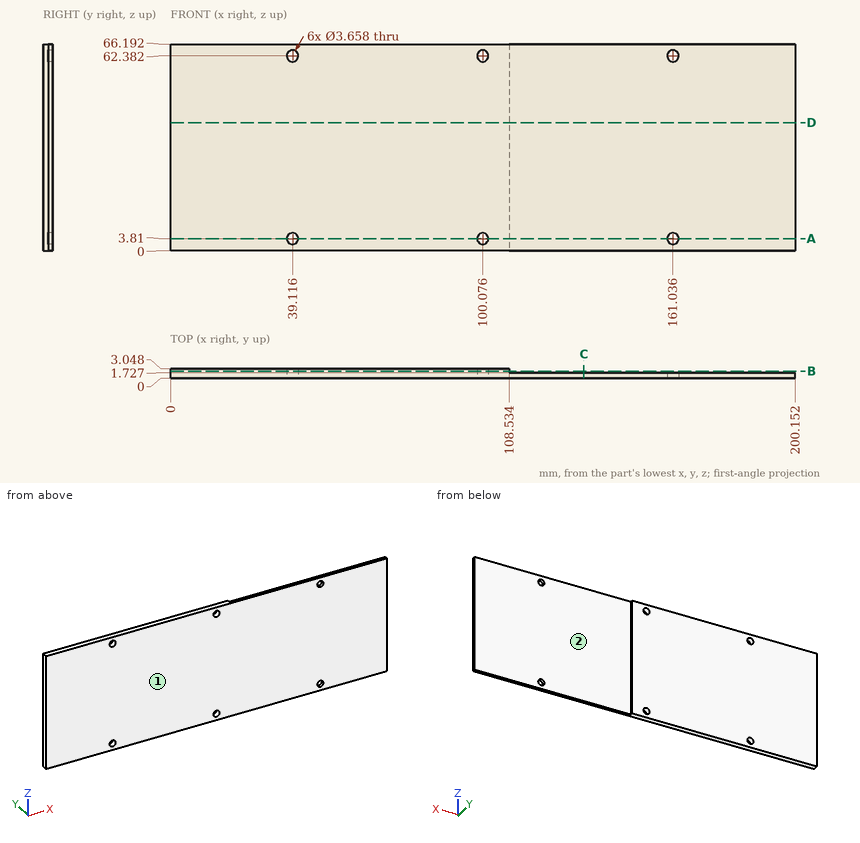
Drawing for the job (mm, zero at the part's lowest x, y, z). A direction names the side the tool comes from. Coordinates: 2 decimals unless noted, no trailing zeros. Order: outer loops, then holes, each group sorted by start corner. A loop starts at its lowest first (then second) coordinate and runs counter-clockwise, first axis right, second up. Notation, with made-up numbers: (17, 39) -> (40, 39) arc R31 cw to (40, 65) -> close; hole circle Ø7 at (6.5, -39.75). An arc over 180 degrees is marked (long way). Return JSON: item names as keys, results as strings.
Item 1: 3-axis set-ups, long thin cutter, end or side, ignore diameter. For the marked faces 1 and 2: which of +Z, -Z, +X, -X, +Y, -Y reach the whole face in a straight line?
Model answer:
{"face 1": "+Z, -Z, +X, -X, -Y", "face 2": "+Z, -Z, +X, +Y"}
Item 2: Wall check: line 1 along X through (y, z) = (0.9, 3.81) (1 decimal); line 2 along X through (y, z) = (1.8, 63) (1 decimal); line 3 along Z through (x, y) = (101.5, 0.35) (1 decimal). Give the ranges that are in metal, low to high. Write a range as from..to.
Model answer:
{"line 1": "x = 0..37.3, 40.9..98.2, 101.9..159.2, 162.9..200.2", "line 2": "x = 0..37.4, 40.8..98.4, 101.8..108.5", "line 3": "z = 0..2.7, 5..61.2, 63.5..66.2"}
Item 3: Slice it at A-A (z = 3.81). Write the cut outline in (x, y) (1 decimal).
Model answer:
{"outline": "(0, 0) -> (37.3, 0) -> (37.3, 3) -> (0, 3) -> close; (40.9, 0) -> (98.2, 0) -> (98.2, 3) -> (40.9, 3) -> close; (101.9, 0) -> (159.2, 0) -> (159.2, 1.7) -> (108.5, 1.7) -> (108.5, 3) -> (101.9, 3) -> close; (162.9, 0) -> (200.2, 0) -> (200.2, 1.7) -> (162.9, 1.7) -> close"}
Item 4: Slice it at C-C (x = 132.5). Write the cut outline in (y, z), then the cut area to 3 significant figures.
Model answer:
{"outline": "(0, 0) -> (1.73, 0) -> (1.73, 66.19) -> (0, 66.19) -> close", "area": "114 mm²"}
Item 5: Slice it at B-B (y = 2.2). Write the cut outline in (x, z) (1 decimal), then the cut area to 3 significant figures.
Model answer:
{"outline": "(0, 0) -> (108.5, 0) -> (108.5, 66.2) -> (0, 66.2) -> close; hole circle Ø3.7 at (39.1, 3.8); hole circle Ø3.7 at (39.1, 62.4); hole circle Ø3.7 at (100.1, 3.8); hole circle Ø3.7 at (100.1, 62.4)", "area": "7,140 mm²"}
Item 6: Pin check, flat tips, straight feed: P1, Ø1, axis at y = 2, z = 45.5, coming from the +X side; P2, Ø6, axis at x = 161.04, z = 62.38, coming from the +Y side; P3, Ø3, axis at x = 100.08, z = 62.38, coming from the -Y side; P4, Ø1.1, axis at y = 2.5, z = 23, coming from the +X side. Stop position of each tip, or through.
Model answer:
{"P1": "stops at x = 200.15", "P2": "stops at y = 1.73", "P3": "passes through", "P4": "stops at x = 108.53"}
Item 7: Slice it at D-D (z = 41). Write the cut outline in (x, y) (1 decimal).
Model answer:
{"outline": "(0, 0) -> (200.2, 0) -> (200.2, 1.7) -> (108.5, 1.7) -> (108.5, 3) -> (0, 3) -> close"}
